```python
from build123d import *

# Parameters (mm, degrees)
SKETCH7_W           = 5.08
SKETCH7_H           = 5.08
BOSS_EXTRUDE3_DEPTH = 17.78
SKETCH8_R           = 1.2065
CUT_EXTRUDE1_DEPTH  = 5.08
FILLET1_R           = 0.254
SKETCH11_R          = 1.905
CUT_EXTRUDE2_DEPTH  = 5.08


with BuildPart() as part:
    # Sketch7 → Boss-Extrude3 (new body)
    with BuildSketch(Plane.XY):
        with Locations((2.448966181, 0.143745058)):
            Rectangle(SKETCH7_W, SKETCH7_H)
    boss_extrude3 = extrude(amount=BOSS_EXTRUDE3_DEPTH)

    # Sketch8 → Cut-Extrude1 (cut)
    with BuildSketch(Plane(origin=(0, 2.683745058, 0), x_dir=(1, 0, 0), z_dir=(0, 1, 0))):
        with Locations(Location((2.448966181, -14.859, 0), (0, 0, 270))):
            Circle(SKETCH8_R)
    cut_extrude1 = extrude(amount=-CUT_EXTRUDE1_DEPTH, mode=Mode.SUBTRACT)

    # Mirror2: Boss-Extrude3, Cut-Extrude1 across plane
    add(boss_extrude3.mirror(Plane.XY))
    add(cut_extrude1.mirror(Plane.XY), mode=Mode.SUBTRACT)

    # Fillet1
    fillet1_edges = [part.edges().sort_by_distance(p)[0] for p in [
        (-0.091033819, 2.683745058, 0),
        (4.988966181, 2.683745058, 0),
        (4.988966181, -2.396254942, 0),
        (-0.091033819, -2.396254942, 0),
    ]]
    fillet(fillet1_edges, radius=FILLET1_R)

    # Sketch11 → Cut-Extrude2 (cut)
    with BuildSketch(Plane.ZY.offset(0.091033819)):
        with Locations(Location((0, 0.143745058, 0), (0, 0, 270))):
            Circle(SKETCH11_R)
    extrude(amount=-CUT_EXTRUDE2_DEPTH, mode=Mode.SUBTRACT)


solid = part.part
```
Read the model definition and answer for the solid it produces. Units are mm, in the model's axes. Coordinates: 2 decimals unless noted, no trailing zeros. Write each loop counter-clockwise with the first axis right and the second up, starting at its lowest first coordinate (ties: lowest second). Pieces come first, ordered by that corner, then holes. Notation, with made-up numbers: (5, 38) -> (11, 38) arc R21 ccw to (11, 71) -> close; hole circle Ø6 at (49.5, 15.25). An arc over 180 degrees is marked (long way). Answer as a JSON object with one key per item and string values.
Q1. The part is cut by section B-B on z = 0. Give the vertices of the cut face in (x, y), then the cut area to 3 significant figures.
The answers:
{"outline": "(-0.09, -2.14) arc R0.25 ccw to (0.16, -2.4) -> (4.73, -2.4) arc R0.25 ccw to (4.99, -2.14) -> (4.99, -1.76) -> (-0.09, -1.76) -> close; (-0.09, 2.05) -> (4.99, 2.05) -> (4.99, 2.43) arc R0.25 ccw to (4.73, 2.68) -> (0.16, 2.68) arc R0.25 ccw to (-0.09, 2.43) -> close", "area": "6.40 mm2"}
Q2. The part is cut by section A-A on x = 3.35. Give the vertices of the cut face in (y, z) (3 decimals), then the cut area to 3 significant figures.
The answers:
{"outline": "(-2.396, -17.78) -> (2.684, -17.78) -> (2.684, -15.661) -> (-2.396, -15.661) -> close; (-2.396, -14.057) -> (2.684, -14.057) -> (2.684, 14.057) -> (-2.396, 14.057) -> close; (-2.396, 15.661) -> (2.684, 15.661) -> (2.684, 17.78) -> (-2.396, 17.78) -> close; hole circle Ø3.81 at (0.144, 0)", "area": "153 mm2"}
Q3. Determine the mould class of faces 1 (the cylindrical face through (2.81, 0.18, 16.01)), 2 (the flat face through (2, -2.396, 0)), 3 (the cylindrical face through (2.41, 0.39, 1.89)), 4 (the flat face through (2, 2.684, 0)) for opening direction Y: pulls with the +Y half, pulls with the -Y half, needs draft (parallel to the pull), parting line crosses it, or undercut.
The answers:
{"face 1": "needs draft", "face 2": "pulls with the -Y half", "face 3": "undercut", "face 4": "pulls with the +Y half"}
Q4. Consider line 1 (Z direction, x = 4, y = 0.3); line 2 (Z direction, x = 1.6, y = -1.2); line 3 (Z direction, x = 3.1, y = 0.4). Determine where each line is inside the solid, lowest interval first. Write a range as [from, to].
The answers:
{"line 1": "z = [-17.78, -1.9], [1.9, 17.78]", "line 2": "z = [-17.78, -15.72], [-14, -1.35], [1.35, 14], [15.72, 17.78]", "line 3": "z = [-17.78, -15.87], [-13.84, -1.89], [1.89, 13.84], [15.87, 17.78]"}
Q5. The part is cut by section C-C on y = 0.7. Give the vertices of the cut face in (x, z), then the cut area to 3 significant figures.
The answers:
{"outline": "(-0.09, -17.78) -> (4.99, -17.78) -> (4.99, -1.82) -> (-0.09, -1.82) -> close; (-0.09, 1.82) -> (4.99, 1.82) -> (4.99, 17.78) -> (-0.09, 17.78) -> close; hole circle Ø2.41 at (2.45, -14.86); hole circle Ø2.41 at (2.45, 14.86)", "area": "153 mm2"}
Q6. The part is cut by section D-D on x = 1.7. Give the vertices of the cut face in (y, z) (3 decimals).
The answers:
{"outline": "(-2.396, -17.78) -> (2.684, -17.78) -> (2.684, -15.805) -> (-2.396, -15.805) -> close; (-2.396, -13.913) -> (2.684, -13.913) -> (2.684, 13.913) -> (-2.396, 13.913) -> close; (-2.396, 15.805) -> (2.684, 15.805) -> (2.684, 17.78) -> (-2.396, 17.78) -> close; hole circle Ø3.81 at (0.144, 0)"}
